```python
from build123d import *

# Parameters (mm, degrees)
F1_DEPTH = 2
F0_R     = 5
F2_DEPTH = 1


with BuildPart() as f1:
    # F0 (on Front) → F1 (new body, symmetric)
    with BuildSketch(Plane.XZ):
        with BuildLine():
            ThreePointArc((-16.772187, 44.440339), (-27.919799, 38.428307), (-37.082383, 29.684118))
            ThreePointArc((-37.082383, 29.684118), (-45.175185, 14.678307), (-47.448165, -2.218477))
            ThreePointArc((-47.448165, -2.218477), (-45.175185, -14.678307), (-39.69036, -26.094546))
            ThreePointArc((-39.69036, -26.094546), (-27.919799, -38.428307), (-12.552392, -45.811434))
            ThreePointArc((-12.552392, -45.811434), (0, -47.5), (12.552392, -45.811434))
            ThreePointArc((12.552392, -45.811434), (27.919799, -38.428307), (39.69036, -26.094546))
            ThreePointArc((39.69036, -26.094546), (45.175185, -14.678307), (47.448165, -2.218477))
            ThreePointArc((47.448165, -2.218477), (45.175185, 14.678307), (37.082383, 29.684118))
            ThreePointArc((37.082383, 29.684118), (27.919799, 38.428307), (16.772187, 44.440339))
            ThreePointArc((16.772187, 44.440339), (0, 47.5), (-16.772187, 44.440339))
        make_face()
    extrude(amount=F1_DEPTH, both=True)

    # F0 (on Front) → F2 (join, symmetric)
    with BuildSketch(Plane.XZ):
        with BuildLine():
            ThreePointArc((-52.142733, 25.729399), (-55.756082, 25.421938), (-58.211244, 22.753044))
            ThreePointArc((-58.211244, 22.753044), (-59.441032, 19.313562), (-60.46779, 15.808112))
            ThreePointArc((-60.46779, 15.808112), (-60.050258, 12.205823), (-57.307718, 9.833209))
            ThreePointArc((-57.307718, 9.833209), (-50.70048, 5.179707), (-47.448165, -2.218477))
            ThreePointArc((-47.448165, -2.218477), (-45.175185, 14.678307), (-37.082383, 29.684118))
            ThreePointArc((-37.082383, 29.684118), (-44.062105, 25.610523), (-52.142733, 25.729399))
        make_face()
        with Locations((-52.308108, 16.995935)):
            Circle(F0_R, mode=Mode.SUBTRACT)
        with BuildLine():
            ThreePointArc((-8.357121, 57.541508), (-10.741116, 49.819639), (-16.772187, 44.440339))
            ThreePointArc((-16.772187, 44.440339), (0, 47.5), (16.772187, 44.440339))
            ThreePointArc((16.772187, 44.440339), (10.741116, 49.819639), (8.357121, 57.541508))
            ThreePointArc((8.357121, 57.541508), (6.948123, 60.882996), (3.651167, 62.393261))
            ThreePointArc((3.651167, 62.393261), (0, 62.5), (-3.651167, 62.393261))
            ThreePointArc((-3.651167, 62.393261), (-6.948123, 60.882996), (-8.357121, 57.541508))
        make_face()
        with Locations((0, 55)):
            Circle(F0_R, mode=Mode.SUBTRACT)
        with BuildLine():
            ThreePointArc((52.142733, 25.729399), (44.062105, 25.610523), (37.082383, 29.684118))
            ThreePointArc((37.082383, 29.684118), (45.175185, 14.678307), (47.448165, -2.218477))
            ThreePointArc((47.448165, -2.218477), (50.70048, 5.179707), (57.307718, 9.833209))
            ThreePointArc((57.307718, 9.833209), (60.050258, 12.205823), (60.46779, 15.808112))
            ThreePointArc((60.46779, 15.808112), (59.441032, 19.313562), (58.211244, 22.753044))
            ThreePointArc((58.211244, 22.753044), (55.756082, 25.421938), (52.142733, 25.729399))
        make_face()
        with Locations((52.308108, 16.995935)):
            Circle(F0_R, mode=Mode.SUBTRACT)
        with BuildLine():
            ThreePointArc((39.69036, -26.094546), (27.919799, -38.428307), (12.552392, -45.811434))
            ThreePointArc((12.552392, -45.811434), (20.593504, -46.618404), (27.060996, -51.46425))
            ThreePointArc((27.060996, -51.46425), (30.164977, -53.339382), (33.719982, -52.62331))
            ThreePointArc((33.719982, -52.62331), (36.736578, -50.563562), (39.627695, -48.331106))
            ThreePointArc((39.627695, -48.331106), (41.407277, -45.171374), (40.583103, -41.639865))
            ThreePointArc((40.583103, -41.639865), (37.972994, -33.991465), (39.69036, -26.094546))
        make_face()
        with Locations((32.328189, -44.495935)):
            Circle(F0_R, mode=Mode.SUBTRACT)
        with BuildLine():
            ThreePointArc((-12.552392, -45.811434), (-27.919799, -38.428307), (-39.69036, -26.094546))
            ThreePointArc((-39.69036, -26.094546), (-37.972994, -33.991465), (-40.583103, -41.639865))
            ThreePointArc((-40.583103, -41.639865), (-41.407277, -45.171374), (-39.627695, -48.331106))
            ThreePointArc((-39.627695, -48.331106), (-36.736578, -50.563562), (-33.719982, -52.62331))
            ThreePointArc((-33.719982, -52.62331), (-30.164977, -53.339382), (-27.060996, -51.46425))
            ThreePointArc((-27.060996, -51.46425), (-20.593504, -46.618404), (-12.552392, -45.811434))
        make_face()
        with Locations((-32.328189, -44.495935)):
            Circle(F0_R, mode=Mode.SUBTRACT)
    extrude(amount=F2_DEPTH, both=True)


solid = f1.part
```
Can you work these out from the model? Positions are in its coordinate system, mm. A direction names the side the tool comes from. Round coordinates to 2 decimals unless told otherwise and drop trailing zeros. Loops run counter-clockwise (first coordinate to the right, second up) from the corner with the lowest first, then second, coordinate; pieces in that order, holes last. Notation, with made-up numbers: (-14, 87) -> (16, 87) arc R32 cw to (16, 123) -> close; hole circle Ø2 at (-40, 15.25). An arc over 180 degrees is marked (long way). One line per item, written item: value. Start each with the question number.
1. If we section it at A-A, the plane x = 0: Write out the boundary of the cut face in (y, z).
2. If we section it at C-C, the plane y = 0.3: Give the number of separate pieces and of enclosed holes in the cut face, then the cut area to 3 significant figures.
3. If we section it at D-D, the plane x = 32: Write out the boundary of the cut face in (y, z), then the cut area to 3 significant figures.
4. For pin 1 (13.5 mm diameter, centred on x = 28.5, z = -40, fed in from -Y); pin 2 (8 mm diameter, centred on x = 32.33, z = -44.5, fed in from -Y); pin 3 (13 mm diameter, centred on x = 52.31, z = 17, fed in from -Y); pin 4 (1 mm diameter, centred on x = -12, y = -0.5, fed in from +Z), each with a flat end and sliding along its axis, tell me the tip position at first contact or that it passes through.
5. If we section it at B-B, the plane z = 55: Write out the boundary of the cut face in (x, y).
6. If we mould it in two halves opening along X, with no side actions, what happens to faces 1 (the cylindrical face through (-43.95, 0.01, 25.64)), 2 (the cylindrical face through (60.026, 0.014, 12.16)), 3 (the flat face through (-28, -1, -41))? For each: pulls with the +X half, pulls with the -X half, needs draft (parallel to the pull), parting line crosses it, or undercut.
7. For faces 4 (the flat face through (-28, 1, -41)), 5 (the flat face through (30.1, 1, -39.7)), 6 (the cylindrical face through (-50.8, 0, 5.3)), 7 (the cylindrical face through (10.803, 0.014, 49.724)), 8 (the cylindrical face through (0.2, 1.5, 47.5)), which set-ups out of +Z, -Z, +X, -X, +Y, -Y let a thin tool reach every point of the face, with its end or its side?
8. If I drill on probe 1 along Z at (x, y) = (-50, 0.4); probe 2 along Y at (x, z) = (27.5, -48); probe 3 along Z at (x, y) = (21, 0.95), over which ranges is the centre line in solid material (lowest first)?
Calculated:
1. outline: (-2, -47.5) -> (2, -47.5) -> (2, 47.5) -> (1, 47.5) -> (1, 50) -> (-1, 50) -> (-1, 47.5) -> (-2, 47.5) -> close; (-1, 60) -> (1, 60) -> (1, 62.5) -> (-1, 62.5) -> close
2. separate pieces: 1
2. enclosed holes: 5
2. area: 8,120 mm²
3. outline: (-2, -35.1) -> (-1, -35.1) -> (-1, -39.51) -> (1, -39.51) -> (1, -35.1) -> (2, -35.1) -> (2, 35.1) -> (-2, 35.1) -> close; (-1, -53.32) -> (1, -53.32) -> (1, -49.49) -> (-1, -49.49) -> close
3. area: 297 mm²
4. pin 1: stops at y = -2
4. pin 2: passes through
4. pin 3: stops at y = -1
4. pin 4: stops at z = 48.74
5. outline: (-8.65, -1) -> (-5, -1) -> (-5, 1) -> (-8.65, 1) -> close; (5, -1) -> (8.65, -1) -> (8.65, 1) -> (5, 1) -> close
6. face 1: undercut
6. face 2: pulls with the +X half
6. face 3: needs draft
7. face 4: -Z, -X, +Y
7. face 5: -Z, +X, +Y
7. face 6: -Z, -X, +Y, -Y
7. face 7: +Z, +X, +Y, -Y
7. face 8: +Z, +Y
8. probe 1: z = 4.25 to 12.56, 21.43 to 25.27
8. probe 2: y = -1 to 1
8. probe 3: z = -46.78 to 42.61
